from build123d import *

# Parameters (mm, degrees)
SKETCH1_W           = 10
SKETCH1_H           = 0.2
BOSS_EXTRUDE1_DEPTH = 10
SKETCH2_R           = 0.150013962
SKETCH2_W           = 0.829232584
SKETCH2_H           = 1.424301619
SKETCH2_W_2         = 1.576755533
SKETCH2_H_2         = 0.841304981
CUT_EXTRUDE1_DEPTH  = 0.1


with BuildPart() as part:
    # Sketch1 → Boss-Extrude1 (new body)
    with BuildSketch(Plane.XY):
        Rectangle(SKETCH1_W, SKETCH1_H)
    extrude(amount=BOSS_EXTRUDE1_DEPTH)

    # Sketch2 → Cut-Extrude1 (cut)
    with BuildSketch(Plane(origin=(0, 0.1, 0), x_dir=(1, 0, 0), z_dir=(0, 1, 0))):
        with Locations(Location((3.903958112, -0.58843737, 0), (0, 0, 180))):
            Circle(SKETCH2_R)
        with Locations(Location((2.904028968, -0.600341426, 0), (0, 0, 180))):
            Circle(SKETCH2_R)
        with Locations(Location((1.904099824, -0.612245481, 0), (0, 0, 180))):
            Circle(SKETCH2_R)
        with Locations(Location((0.904170679, -0.624149537, 0), (0, 0, 180))):
            Circle(SKETCH2_R)
        with Locations(Location((-0.095758465, -0.636053593, 0), (0, 0, 180))):
            Circle(SKETCH2_R)
        with Locations(Location((-1.095687609, -0.647957649, 0), (0, 0, 180))):
            Circle(SKETCH2_R)
        with Locations(Location((-2.095616753, -0.659861704, 0), (0, 0, 180))):
            Circle(SKETCH2_R)
        with Locations(Location((-3.095545897, -0.67176576, 0), (0, 0, 180))):
            Circle(SKETCH2_R)
        with Locations(Location((-4.095475042, -0.683669816, 0), (0, 0, 180))):
            Circle(SKETCH2_R)
        with Locations((-4.095475042, -9.395473292)):
            Circle(SKETCH2_R)
        with Locations((-3.095545897, -9.407377347)):
            Circle(SKETCH2_R)
        with Locations((-2.095616753, -9.419281403)):
            Circle(SKETCH2_R)
        with Locations((-1.095687609, -9.431185459)):
            Circle(SKETCH2_R)
        with Locations((0.904170679, -9.45499357)):
            Circle(SKETCH2_R)
        with Locations((-0.095758465, -9.443089515)):
            Circle(SKETCH2_R)
        with Locations((1.904099824, -9.466897626)):
            Circle(SKETCH2_R)
        with Locations((2.904028968, -9.478801682)):
            Circle(SKETCH2_R)
        with Locations((3.903958112, -9.490705738)):
            Circle(SKETCH2_R)
        Polygon((1.476108968, -4.618919063), (0.189761323, -3.332571418), (-1.096586323, -4.618919063), (0.189761323, -5.905266709), align=None)
        with Locations((-3.012916665, -4.618919063)):
            Rectangle(SKETCH2_W, SKETCH2_H)
        with Locations((2.806863526, -4.618919063)):
            Rectangle(SKETCH2_W_2, SKETCH2_H_2)
    extrude(amount=-CUT_EXTRUDE1_DEPTH, mode=Mode.SUBTRACT)


solid = part.part
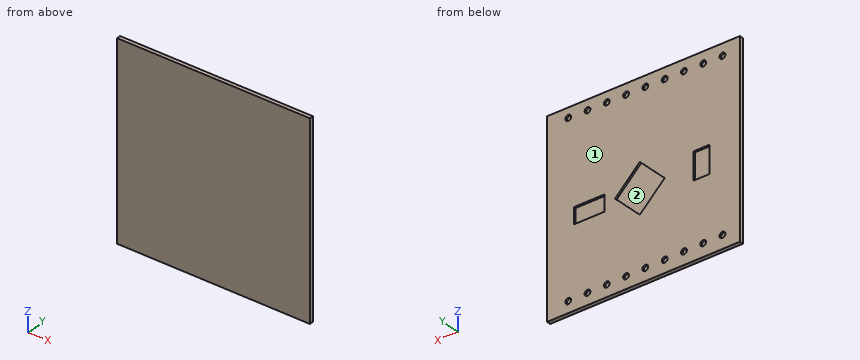
Source: CAD feature listing. Evaluate the final solid. Frame: model axes, mm. Face numbers are marked on the shaded views. Give positions to 0.01 mm unless a question says otherwise; leave off trailing zeros. Order: outer loops, then holes, each group sorted by start corner. A loop starts at its lowest first (then second) coordinate and runs counter-clockwise, first axis right, second up. Notation, with made-up numbers: (-17, 53.5) -> (26, 53.5) arc R17 ccw to (26, 77.5) -> close; hole circle Ø8 at (-34.75, -8). An arc over 180 degrees is marked (long way). Use a Markdown table: item, result.
1) Mould query, pull axis X, two halves, no side actions, for the marked faces 1 and 2. Classes: +X half, -X half, draft (parallel to the pull), parting line (faces both ways), or undercut.
Answer list:
| item | result |
|---|---|
| face 1 | draft |
| face 2 | undercut |
2) Section query B-B, the plane x = -2.75. Return the cut outline in (y, z), then the cut area to 3 significant figures.
Answer list:
| item | result |
|---|---|
| outline | (-0.1, 0) -> (0.1, 0) -> (0.1, 3.91) -> (0, 3.91) -> (0, 5.33) -> (0.1, 5.33) -> (0.1, 10) -> (-0.1, 10) -> close |
| area | 1.86 mm² |
3) Ray query, line 1 along Z through (x, y) = (-0.5, 0.05); line 2 along X through (y, z) = (0.05, 3.75). Return the intervals inside material, ascending. Write a range as [from, to].
Answer list:
| item | result |
|---|---|
| line 1 | [0, 4.02], [5.22, 10] |
| line 2 | [-5, -0.23], [0.61, 5] |
4) Contact query for a flat-ended pin moving along its axis: P1, Ø0.7, axis at x = -3, z = 4.5, coming from the +Y side. Output: stop coordinate, or through.
Answer list:
| item | result |
|---|---|
| P1 | y = 0 |
5) Section query C-C, the plane z = 4.5. Return the cut outline in (x, y).
Answer list:
| item | result |
|---|---|
| outline | (-5, -0.1) -> (5, -0.1) -> (5, 0.1) -> (3.6, 0.1) -> (3.6, 0) -> (2.02, 0) -> (2.02, 0.1) -> (1.36, 0.1) -> (1.36, 0) -> (-0.98, 0) -> (-0.98, 0.1) -> (-2.6, 0.1) -> (-2.6, 0) -> (-3.43, 0) -> (-3.43, 0.1) -> (-5, 0.1) -> close |
6) Section query A-A, the plane x = 2.25. Return the cut outline in (y, z).
Answer list:
| item | result |
|---|---|
| outline | (-0.1, 0) -> (0.1, 0) -> (0.1, 4.2) -> (0, 4.2) -> (0, 5.04) -> (0.1, 5.04) -> (0.1, 10) -> (-0.1, 10) -> close |
